Source: CAD feature listing. Evaluate the final solid. Frame: model axes, mm. A direction names the side the tool comes from. Coordinates: 2 decimals unless noted, no trailing zeros. Write each loop counter-clockwise with the first axis right and the second up, starting at its lowest first coordinate (ties: lowest second). Pieces come first, ordered by that corner, then holes. Notation, with made-up numbers: (-23, 19.25) - (21, 19.25) arc R21 ccw to (21, 40.25) - close; hole circle Ø2 at (30, 45.25). An arc over 180 degrees is marked (long way). One line per question, with ' | ' between items. Start each with the question number.
Q1. Line query: line 1 (Z direction, x = 10.5, y = 1.75); line 2 (Z direction, x = 0.5, y = -17.5); line 3 (X direction, y = -1, z = -45). Output: solid intervals per line, ascending.
Q2. Contact query for a flat-ended pin moving along its axis: P1, Ø10.5, axis at y = -7, z = 14.5, coming from the +X side. Output: stop coordinate, or through.
Q3. Cut plane A-A, the plane z = -36.5. Return loops of the section in (x, y), plus the area to 3 significant figures.
Q4. Cut plane D-D, the plane y = -14.5. Return loops of the section in (x, z), plus the area to 3 significant figures.
Q5. Cut plane B-B, the plane y = -10.5. Return loops of the section in (x, z), plus the area to 3 significant figures.
Q6. Cut plane C-C, the plane x = 10.5. Return loops of the section in (y, z), plus the area to 3 significant figures.
Q7. Draft query along Z for faces 1 (the face through (10.142, 1.479, 39.227)), 2 (the face through (7, -6, -50)), 3 (the face through (9, 3, 1)). Return one class per face: +Z half, -Z half, draft (parallel to the pull), parting line (faces both ways), or undercut.
Q8. Access query for faces 4 (the face through (-3, -9, 1)), 5 (the face through (0, -11, 1)). Directions: +Z, -Z, +X, -X, +Y, -Y. A direction counts if a zero-diameter tool reaches every point of the face in a straight line with its end or side. Return the directions, or none.
```python
from build123d import *

# Parameters (mm, degrees)
PAD_DEPTH     = 50
SKETCH001_W   = 24
SKETCH001_H   = 24
POCKET_DEPTH  = 47
SKETCH002_R   = 2.75
HOLE_DEPTH    = 3.001
SKETCH003_R   = 2.75
HOLE001_DEPTH = 3.001


with BuildPart() as part:
    # Sketch → Pad (new body, symmetric)
    with BuildSketch(Plane.XY):
        Polygon((-3, 3), (21, 3), (21, 0), (0, -21), (-3, -21), align=None)
    extrude(amount=PAD_DEPTH, both=True)

    # Sketch001 → Pocket (cut, symmetric)
    with BuildSketch(Plane.XY):
        with Locations((12, -12)):
            Rectangle(SKETCH001_W, SKETCH001_H)
    extrude(amount=POCKET_DEPTH, both=True, mode=Mode.SUBTRACT)

    # Sketch002 → Hole (cut, through all)
    with BuildSketch(Plane.YZ):
        with Locations((-10.5, 36.5)):
            Circle(SKETCH002_R)
        with Locations((-10.5, -36.5)):
            Circle(SKETCH002_R)
    extrude(amount=-HOLE_DEPTH, mode=Mode.SUBTRACT)

    # Sketch003 → Hole001 (cut, through all)
    with BuildSketch(Plane.XZ):
        with Locations((10.5, 36.5)):
            Circle(SKETCH003_R)
        with Locations((10.5, -36.5)):
            Circle(SKETCH003_R)
    extrude(amount=-HOLE001_DEPTH, mode=Mode.SUBTRACT)


solid = part.part
```
Reply:
1) line 1: z = -50 to -39.25, -33.75 to 33.75, 39.25 to 50 | line 2: z = -50 to -47, 47 to 50 | line 3: x = -3 to 0
2) P1: stops at x = 0
3) outline: (-3, -21) - (0, -21) - (0, -13.25) - (-3, -13.25) - close; (-3, -7.75) - (0, -7.75) - (0, 0) - (7.75, 0) - (7.75, 3) - (-3, 3) - close; (13.25, 0) - (21, 0) - (21, 3) - (13.25, 3) - close | area: 102 mm^2
4) outline: (-3, -50) - (6.5, -50) - (6.5, -47) - (0, -47) - (0, 47) - (6.5, 47) - (6.5, 50) - (-3, 50) - close | area: 339 mm^2
5) outline: (-3, -50) - (10.5, -50) - (10.5, -47) - (0, -47) - (0, -39.25) - (-3, -39.25) - close; (-3, -33.75) - (0, -33.75) - (0, 33.75) - (-3, 33.75) - close; (-3, 39.25) - (0, 39.25) - (0, 47) - (10.5, 47) - (10.5, 50) - (-3, 50) - close | area: 330 mm^2
6) outline: (-10.5, -50) - (3, -50) - (3, -39.25) - (0, -39.25) - (0, -47) - (-10.5, -47) - close; (-10.5, 47) - (0, 47) - (0, 39.25) - (3, 39.25) - (3, 50) - (-10.5, 50) - close; (0, -33.75) - (3, -33.75) - (3, 33.75) - (0, 33.75) - close | area: 330 mm^2
7) face 1: undercut | face 2: -Z half | face 3: draft
8) face 4: +Z, -Z, -X, +Y, -Y | face 5: +X, -Y
